from build123d import *

# Parameters (mm, degrees)
SKETCH1_R           = 7
BOSS_EXTRUDE1_DEPTH = 2
CUT_EXTRUDE1_REACH  = 12.677
SKETCH2_R           = 3.9
CHAMFER1_SIZE       = 0.5
FILLET1_R           = 0.1


with BuildPart() as part:
    # Sketch1 → Boss-Extrude1 (new, symmetric)
    with BuildSketch(Plane(origin=(0, 0, 0), x_dir=(1, 0, 0), z_dir=(0, 1, 0))):
        with Locations(Location((0, 0, 0), (0, 0, 270))):
            Circle(SKETCH1_R)
    extrude(amount=BOSS_EXTRUDE1_DEPTH, both=True)

    # Sketch2 → Cut-Extrude1 (cut, up to next)
    with BuildSketch(Plane(origin=(0, 2, 0), x_dir=(1, 0, 0), z_dir=(0, 1, 0)), mode=Mode.PRIVATE) as cut_extrude1_sk1:
        with Locations(Location((0, 0, 0), (0, 0, 270))):
            Circle(SKETCH2_R)
    cut_extrude1_tool1 = extrude(cut_extrude1_sk1.sketch, amount=-CUT_EXTRUDE1_REACH, mode=Mode.PRIVATE) & part.part
    add(cut_extrude1_tool1.solids().sort_by_distance((0, 2, 0))[0], mode=Mode.SUBTRACT)

    # Chamfer1
    chamfer1_edges = [part.edges().sort_by_distance(p)[0] for p in [
        (0, -2, -3.9),
    ]]
    chamfer(chamfer1_edges, length=CHAMFER1_SIZE)

    # Fillet1
    fillet1_edges = [part.edges().sort_by_distance(p)[0] for p in [
        (0, -2, -7),
        (0, 2, -7),
    ]]
    fillet(fillet1_edges, radius=FILLET1_R)


solid = part.part
Check sheet for the modelled part. Datum: model origin and axes. Units: mm. Give positions to 0.01 mm unless a question says otherwise; leave off trailing zeros. Loops run counter-clockwise (first coordinate to the right, second up) from the corner with the lowest first, then second, coordinate; pieces in that order, holes last. Notation, with made-up numbers: M -40,63 L -17,63 A20 ccw -17,82 Z; hole C 21.5,83.25 d7. An arc over 180 degrees is marked long. Return JSON: item names as keys, results as strings. Group by question number.
1. Mould release check, pull along X, two halves, no side actions. Record for faces 1 (the cylindrical face through (-6.834, 0.027, -1.517)), 2 (the cylindrical face through (-2.373, 0.274, -3.095)), 3 (the flat face through (-5, -2, 0)): released by +X, released by -X, zero draft, split by the parting line, or undercut.
2. Go/stop test with flat-tipped pins: pin 1 (1.5 mm diameter, centred on y = -1, z = -4.5, fed in from +X); pin 2 (1 mm diameter, centred on x = 5, y = -1.5, fed in from -Z). Record where each tip stops, or that it passes through.
3. Cross-section at B-B on z = 0. Record the boundary of the cut face in (x, y), plus the area to 3 significant figures.
4. Cross-section at A-A on x = 0. Record the boundary of the cut face in (y, z).
5. Cross-section at C-C on y = -0.85. Record the boundary of the cut face in (x, z), plus the area to 3 significant figures.
6. Thickness scan on L1, parallel to X at y = 0, z = 0; L2, parallel to Z at x = -1.5, y = 0; L3, parallel to X at y = -1.55, z = 1.5. Record the ranges inside material, lowest first.
Return value:
{
 "1": {"face 1": "split by the parting line", "face 2": "undercut", "face 3": "zero draft"},
 "2": {"pin 1": "x = 5.91", "pin 2": "z = -5.36"},
 "3": {"outline": "M -7,-1.9 A0.1 ccw -6.9,-2 L -4.4,-2 L -3.9,-1.5 L -3.9,2 L -6.9,2 A0.1 ccw -7,1.9 Z; M 3.9,-1.5 L 4.4,-2 L 6.9,-2 A0.1 ccw 7,-1.9 L 7,1.9 A0.1 ccw 6.9,2 L 3.9,2 Z", "area": "24.5 mm^2"},
 "4": {"outline": "M -2,-6.9 A0.1 ccw -1.9,-7 L 1.9,-7 A0.1 ccw 2,-6.9 L 2,-3.9 L -1.5,-3.9 L -2,-4.4 Z; M -2,4.4 L -1.5,3.9 L 2,3.9 L 2,6.9 A0.1 ccw 1.9,7 L -1.9,7 A0.1 ccw -2,6.9 Z"},
 "5": {"outline": "C 0,0 d14; hole C 0,0 d7.8", "area": "106 mm^2"},
 "6": {"L1": "-7 to -3.9, 3.9 to 7", "L2": "-6.84 to -3.6, 3.6 to 6.84", "L3": "-6.84 to -3.65, 3.65 to 6.84"}
}
